The listing builds one solid part. Answer for the finished solid, in the listing's coordinates (mm). A direction names the side the tool comes from. Give positions to 0.01 mm unless a question says otherwise; leave off trailing zeros. Write each loop counter-clockwise with the first axis right and the second up, starting at its lowest first coordinate (ties: lowest second). Pieces come first, ordered by that corner, then holes. Notation, with made-up numbers: M 43.5,63.5 L 62.5,63.5 A15 cw 62.5,75.5 Z; hole C 60.25,73 d10. An arc over 180 degrees is marked long. Answer as a JSON object with one key per item and string values.
```python
from build123d import *

# Parameters (mm, degrees)
SKETCH_1_W                    = 20
SKETCH_1_H                    = 54.5
EXTRUDE_1_DEPTH               = 1
SKETCH_2_W                    = 20
SKETCH_2_H                    = 1
EXTRUDE_2_DEPTH               = 38
SKETCH_3_W                    = 20
SKETCH_3_H                    = 1
EXTRUDE_3_DEPTH               = 38
SKETCH_4_R                    = 4.1
CUT_EXTRUDE_1_DEPTH           = 1
SKETCH_5_R                    = 0.79
CUT_EXTRUDE_2_DEPTH           = 1
SKETCH_6_R                    = 0.79
CUT_EXTRUDE_3_DEPTH           = 1
SKETCH_7_R                    = 0.79
CUT_EXTRUDE_4_DEPTH           = 1
SKETCH_8_R                    = 0.79
CUT_EXTRUDE_5_DEPTH           = 1
SKETCH_9_R                    = 1.6
CUT_EXTRUDE_6_DEPTH           = 1
CUT_EXTRUDE_7_REACH           = 71.937
SKETCH_10_R                   = 1.6
CUT_EXTRUDE_8_REACH           = 71.937
SKETCH_11_R                   = 1.6
CUT_EXTRUDE_9_REACH           = 71.937
SKETCH_12_R                   = 1.6
CUT_EXTRUDE_10_REACH          = 71.937
SKETCH_14_R                   = 1.6
SHEET_START                   = -38
SHEET_METAL_1_OUTLINE_W       = 1
SHEET_METAL_1_OUTLINE_H       = 20
SHEET_METAL_1_DEPTH           = 38
SHEET_METAL_1_2_OUTLINE_W     = 37.35619449
SHEET_METAL_1_2_OUTLINE_H     = 20
SHEET_METAL_1_2_OUTLINE_R     = 0.79
SHEET_METAL_1_2_OUTLINE_R_2   = 4.1
SHEET_METAL_1_2_OUTLINE_R_3   = 1.6
SHEET_METAL_1_2_DEPTH         = 1
SHEET_START_2                 = 54.28876
SHEET_METAL_1_3_OUTLINE_W     = 1
SHEET_METAL_1_3_OUTLINE_H     = 20
SHEET_METAL_1_3_DEPTH         = 37.56743449
SHEET_START_3                 = -37.35619449
SHEET_METAL_1_3_2_OUTLINE_W   = 1
SHEET_METAL_1_3_2_OUTLINE_H   = 20
SHEET_METAL_1_3_2_DEPTH       = 37.55071449
SHEET_METAL_1_3_3_OUTLINE_R   = 4.1
SHEET_METAL_1_3_3_OUTLINE_R_2 = 1.6
SHEET_METAL_1_3_3_OUTLINE_R_3 = 0.79
SHEET_METAL_1_3_3_DEPTH       = 1
SHEET_METAL_1_3_4_OUTLINE_W   = 38
SHEET_METAL_1_3_4_OUTLINE_H   = 20
SHEET_METAL_1_3_4_OUTLINE_R   = 0.79
SHEET_METAL_1_3_4_OUTLINE_R_2 = 4.1
SHEET_METAL_1_3_4_DEPTH       = 2
SHEET_START_4                 = 52.5
SHEET_METAL_1_3_5_OUTLINE_W   = 38
SHEET_METAL_1_3_5_OUTLINE_H   = 20
SHEET_METAL_1_3_5_OUTLINE_R   = 0.79
SHEET_METAL_1_3_5_OUTLINE_R_2 = 4.1
SHEET_METAL_1_3_5_DEPTH       = 2
SHEET_START_5                 = -20
SHEET_METAL_1_3_6_DEPTH       = 20


with BuildPart() as part:
    # Sketch 1 → ﾎﾞｽ - 押し出し1 (new body)
    with BuildSketch(Plane(origin=(0, 0, 0), x_dir=(0, 0, -1), z_dir=(1, 0, 0))):
        with Locations((10, 27.25)):
            Rectangle(SKETCH_1_W, SKETCH_1_H)
    extrude(amount=EXTRUDE_1_DEPTH)

    # Sketch 2 → ﾎﾞｽ - 押し出し2 (add)
    with BuildSketch(Plane.ZY):
        with Locations((-10, 54)):
            Rectangle(SKETCH_2_W, SKETCH_2_H)
    extrude(amount=EXTRUDE_2_DEPTH)

    # ｽｹｯﾁ3 → ﾎﾞｽ - 押し出し3 (add)
    with BuildSketch(Plane.ZY):
        with Locations((-10, 0.5)):
            Rectangle(SKETCH_3_W, SKETCH_3_H)
    extrude(amount=EXTRUDE_3_DEPTH)

    # ｽｹｯﾁ4 → ｶｯﾄ - 押し出し1 (cut)
    with BuildSketch(Plane(origin=(0, 54.5, 0), x_dir=(1, 0, 0), z_dir=(0, 1, 0))):
        with Locations(Location((-26.39, 10, 0), (0, 0, 270))):
            Circle(SKETCH_4_R)
    extrude(amount=-CUT_EXTRUDE_1_DEPTH, mode=Mode.SUBTRACT)

    # ｽｹｯﾁ5 → ｶｯﾄ - 押し出し2 (cut)
    with BuildSketch(Plane(origin=(0, 54.5, 0), x_dir=(1, 0, 0), z_dir=(0, 1, 0))):
        with Locations(Location((-33.88, 10, 0), (0, 0, 270))):
            Circle(SKETCH_5_R)
    extrude(amount=-CUT_EXTRUDE_2_DEPTH, mode=Mode.SUBTRACT)

    # ｽｹｯﾁ6 → ｶｯﾄ - 押し出し3 (cut)
    with BuildSketch(Plane(origin=(0, 54.5, 0), x_dir=(1, 0, 0), z_dir=(0, 1, 0))):
        with Locations(Location((-18.9, 10, 0), (0, 0, 270))):
            Circle(SKETCH_6_R)
    extrude(amount=-CUT_EXTRUDE_3_DEPTH, mode=Mode.SUBTRACT)

    # ｽｹｯﾁ7 → ｶｯﾄ - 押し出し4 (cut)
    with BuildSketch(Plane(origin=(0, 54.5, 0), x_dir=(1, 0, 0), z_dir=(0, 1, 0))):
        with Locations(Location((-26.39, 2.51, 0), (0, 0, 270))):
            Circle(SKETCH_7_R)
    extrude(amount=-CUT_EXTRUDE_4_DEPTH, mode=Mode.SUBTRACT)

    # ｽｹｯﾁ8 → ｶｯﾄ - 押し出し5 (cut)
    with BuildSketch(Plane(origin=(0, 54.5, 0), x_dir=(1, 0, 0), z_dir=(0, 1, 0))):
        with Locations(Location((-26.39, 17.49, 0), (0, 0, 270))):
            Circle(SKETCH_8_R)
    extrude(amount=-CUT_EXTRUDE_5_DEPTH, mode=Mode.SUBTRACT)

    # ｽｹｯﾁ9 → ｶｯﾄ - 押し出し6 (cut)
    with BuildSketch(Plane(origin=(0, 0, 0), x_dir=(-1, 0, 0), z_dir=(0, -1, 0))):
        with Locations(Location((26.39, 10, 0), (0, 0, 90))):
            Circle(SKETCH_9_R)
    extrude(amount=-CUT_EXTRUDE_6_DEPTH, mode=Mode.SUBTRACT)

    # ｽｹｯﾁ10 → ｶｯﾄ - 押し出し7 (cut, up to next)
    with BuildSketch(Plane(origin=(1, 0, 0), x_dir=(0, 0, -1), z_dir=(1, 0, 0)), mode=Mode.PRIVATE) as cut_extrude_7_sk1:
        with Locations((17, 27.25)):
            Circle(SKETCH_10_R)
    cut_extrude_7_tool1 = extrude(cut_extrude_7_sk1.sketch, amount=-CUT_EXTRUDE_7_REACH, mode=Mode.PRIVATE) & part.part
    add(cut_extrude_7_tool1.solids().sort_by_distance((1, 27.25, -17))[0], mode=Mode.SUBTRACT)

    # ｽｹｯﾁ11 → ｶｯﾄ - 押し出し8 (cut, up to next)
    with BuildSketch(Plane(origin=(1, 0, 0), x_dir=(0, 0, -1), z_dir=(1, 0, 0)), mode=Mode.PRIVATE) as cut_extrude_8_sk1:
        with Locations((3, 27.25)):
            Circle(SKETCH_11_R)
    cut_extrude_8_tool1 = extrude(cut_extrude_8_sk1.sketch, amount=-CUT_EXTRUDE_8_REACH, mode=Mode.PRIVATE) & part.part
    add(cut_extrude_8_tool1.solids().sort_by_distance((1, 27.25, -3))[0], mode=Mode.SUBTRACT)

    # ｽｹｯﾁ12 → ｶｯﾄ - 押し出し9 (cut, up to next)
    with BuildSketch(Plane(origin=(1, 0, 0), x_dir=(0, 0, -1), z_dir=(1, 0, 0)), mode=Mode.PRIVATE) as cut_extrude_9_sk1:
        with Locations((10, 23.75)):
            Circle(SKETCH_12_R)
    cut_extrude_9_tool1 = extrude(cut_extrude_9_sk1.sketch, amount=-CUT_EXTRUDE_9_REACH, mode=Mode.PRIVATE) & part.part
    add(cut_extrude_9_tool1.solids().sort_by_distance((1, 23.75, -10))[0], mode=Mode.SUBTRACT)

    # ｽｹｯﾁ14 → ｶｯﾄ - 押し出し10 (cut, up to next)
    with BuildSketch(Plane(origin=(1, 0, 0), x_dir=(0, 0, -1), z_dir=(1, 0, 0)), mode=Mode.PRIVATE) as cut_extrude_10_sk1:
        with Locations((10, 30.75)):
            Circle(SKETCH_14_R)
    cut_extrude_10_tool1 = extrude(cut_extrude_10_sk1.sketch, amount=-CUT_EXTRUDE_10_REACH, mode=Mode.PRIVATE) & part.part
    add(cut_extrude_10_tool1.solids().sort_by_distance((1, 30.75, -10))[0], mode=Mode.SUBTRACT)

    # Sheet Metal 1: read off the stored shape, not the designer's step
    # Sheet Metal 1 outline → Sheet Metal 1 (cut)
    with BuildSketch(Plane.YZ.offset(SHEET_START)):
        with Locations((54, -10)):
            Rectangle(SHEET_METAL_1_OUTLINE_W, SHEET_METAL_1_OUTLINE_H)
        with Locations((0.5, -10)):
            Rectangle(SHEET_METAL_1_OUTLINE_W, SHEET_METAL_1_OUTLINE_H)
    extrude(amount=SHEET_METAL_1_DEPTH, mode=Mode.SUBTRACT)

    # Sheet Metal 1 2 outline → Sheet Metal 1 2 (add)
    # profile 1 of 2: a face of its own
    with BuildSketch(Plane.YZ):
        with Locations((73.178097245, -10)):
            Rectangle(SHEET_METAL_1_2_OUTLINE_W, SHEET_METAL_1_2_OUTLINE_H)
        with Locations((80.24619449, -17.49)):
            Circle(SHEET_METAL_1_2_OUTLINE_R, mode=Mode.SUBTRACT)
        with Locations((72.75619449, -10)):
            Circle(SHEET_METAL_1_2_OUTLINE_R, mode=Mode.SUBTRACT)
        with Locations((80.24619449, -10)):
            Circle(SHEET_METAL_1_2_OUTLINE_R_2, mode=Mode.SUBTRACT)
        with Locations((87.73619449, -10)):
            Circle(SHEET_METAL_1_2_OUTLINE_R, mode=Mode.SUBTRACT)
        with Locations((80.24619449, -2.51)):
            Circle(SHEET_METAL_1_2_OUTLINE_R, mode=Mode.SUBTRACT)
    # profile 2 of 2: a face of its own
    with BuildSketch(Plane.YZ):
        with Locations((-18.678097245, -10)):
            Rectangle(SHEET_METAL_1_2_OUTLINE_W, SHEET_METAL_1_2_OUTLINE_H)
        with Locations((-25.74619449, -10)):
            Circle(SHEET_METAL_1_2_OUTLINE_R_3, mode=Mode.SUBTRACT)
    extrude(amount=SHEET_METAL_1_2_DEPTH)

    # Sheet Metal 1 3: read off the stored shape, not the designer's step
    # Sheet Metal 1 3 outline → Sheet Metal 1 3 (cut)
    with BuildSketch(Plane(origin=(0, 0, 0), x_dir=(1, 0, 0), z_dir=(0, 1, 0)).offset(SHEET_START_2)):
        with Locations((0.5, 10)):
            Rectangle(SHEET_METAL_1_3_OUTLINE_W, SHEET_METAL_1_3_OUTLINE_H)
    extrude(amount=SHEET_METAL_1_3_DEPTH, mode=Mode.SUBTRACT)

    # Sheet Metal 1 3 2 outline → Sheet Metal 1 3 2 (cut)
    with BuildSketch(Plane(origin=(0, 0, 0), x_dir=(1, 0, 0), z_dir=(0, 1, 0)).offset(SHEET_START_3)):
        with Locations((0.5, 10)):
            Rectangle(SHEET_METAL_1_3_2_OUTLINE_W, SHEET_METAL_1_3_2_OUTLINE_H)
    extrude(amount=SHEET_METAL_1_3_2_DEPTH, mode=Mode.SUBTRACT)



with BuildPart() as body_2:
    # Sheet Metal 1 3 3 outline → Sheet Metal 1 3 3 (new body)
    # profile 1 of 5: a face of its own
    with BuildSketch(Plane(origin=(0, 0, 0), x_dir=(1, 0, 0), z_dir=(0, 1, 0))):
        with Locations((-26.39, 10)):
            Circle(SHEET_METAL_1_3_3_OUTLINE_R)
        with Locations((-26.39, 10)):
            Circle(SHEET_METAL_1_3_3_OUTLINE_R_2, mode=Mode.SUBTRACT)
    # profile 2 of 5: a face of its own
    with BuildSketch(Plane(origin=(0, 0, 0), x_dir=(1, 0, 0), z_dir=(0, 1, 0))):
        with Locations((-33.88, 10)):
            Circle(SHEET_METAL_1_3_3_OUTLINE_R_3)
    # profile 3 of 5: a face of its own
    with BuildSketch(Plane(origin=(0, 0, 0), x_dir=(1, 0, 0), z_dir=(0, 1, 0))):
        with Locations((-18.9, 10)):
            Circle(SHEET_METAL_1_3_3_OUTLINE_R_3)
    # profile 4 of 5: a face of its own
    with BuildSketch(Plane(origin=(0, 0, 0), x_dir=(1, 0, 0), z_dir=(0, 1, 0))):
        with Locations((-26.39, 2.51)):
            Circle(SHEET_METAL_1_3_3_OUTLINE_R_3)
    # profile 5 of 5: a face of its own
    with BuildSketch(Plane(origin=(0, 0, 0), x_dir=(1, 0, 0), z_dir=(0, 1, 0))):
        with Locations((-26.39, 17.49)):
            Circle(SHEET_METAL_1_3_3_OUTLINE_R_3)
    extrude(amount=SHEET_METAL_1_3_3_DEPTH)


with BuildPart() as part_1:
    add(part.part)

    add(body_2.part)  # Sheet Metal 1 3 4 merges body 2
    # Sheet Metal 1 3 4 outline → Sheet Metal 1 3 4 (add)
    with BuildSketch(Plane(origin=(0, 0, 0), x_dir=(1, 0, 0), z_dir=(0, 1, 0))):
        with Locations((-19, 10)):
            Rectangle(SHEET_METAL_1_3_4_OUTLINE_W, SHEET_METAL_1_3_4_OUTLINE_H)
        with Locations((-26.39, 2.51)):
            Circle(SHEET_METAL_1_3_4_OUTLINE_R, mode=Mode.SUBTRACT)
        with Locations((-33.88, 10)):
            Circle(SHEET_METAL_1_3_4_OUTLINE_R, mode=Mode.SUBTRACT)
        with Locations((-26.39, 10)):
            Circle(SHEET_METAL_1_3_4_OUTLINE_R_2, mode=Mode.SUBTRACT)
        with Locations((-18.9, 10)):
            Circle(SHEET_METAL_1_3_4_OUTLINE_R, mode=Mode.SUBTRACT)
        with Locations((-26.39, 17.49)):
            Circle(SHEET_METAL_1_3_4_OUTLINE_R, mode=Mode.SUBTRACT)
    extrude(amount=SHEET_METAL_1_3_4_DEPTH)

    # Sheet Metal 1 3 5 outline → Sheet Metal 1 3 5 (add)
    with BuildSketch(Plane(origin=(0, 0, 0), x_dir=(1, 0, 0), z_dir=(0, 1, 0)).offset(SHEET_START_4)):
        with Locations((-19, 10)):
            Rectangle(SHEET_METAL_1_3_5_OUTLINE_W, SHEET_METAL_1_3_5_OUTLINE_H)
        with Locations((-26.39, 2.51)):
            Circle(SHEET_METAL_1_3_5_OUTLINE_R, mode=Mode.SUBTRACT)
        with Locations((-33.88, 10)):
            Circle(SHEET_METAL_1_3_5_OUTLINE_R, mode=Mode.SUBTRACT)
        with Locations((-26.39, 10)):
            Circle(SHEET_METAL_1_3_5_OUTLINE_R_2, mode=Mode.SUBTRACT)
        with Locations((-18.9, 10)):
            Circle(SHEET_METAL_1_3_5_OUTLINE_R, mode=Mode.SUBTRACT)
        with Locations((-26.39, 17.49)):
            Circle(SHEET_METAL_1_3_5_OUTLINE_R, mode=Mode.SUBTRACT)
    extrude(amount=SHEET_METAL_1_3_5_DEPTH)

    # Sheet Metal 1 3 6 outline → Sheet Metal 1 3 6 (cut)
    with BuildSketch(Plane.XY.offset(SHEET_START_5)):
        with BuildLine():
            Line((-38, 2), (-38, 1))
            Line((-38, 1), (-1, 1))
            ThreePointArc((-1, 1), (-0.292893219, 1.292893219), (0, 2))
            Line((0, 2), (-38, 2))
        make_face()
        with BuildLine():
            Line((-1, 53.5), (-38, 53.5))
            Line((-38, 53.5), (-38, 52.5))
            Line((-38, 52.5), (0, 52.5))
            ThreePointArc((0, 52.5), (-0.292893219, 53.207106781), (-1, 53.5))
        make_face()
        with BuildLine():
            ThreePointArc((-1, 54.5), (0.414213562, 53.914213562), (1, 52.5))
            Line((1, 52.5), (1, 54.28876))
            Line((1, 54.28876), (0, 54.28876))
            Line((0, 54.28876), (0, 54.5))
            Line((0, 54.5), (-1, 54.5))
        make_face()
        with BuildLine():
            ThreePointArc((1, 2), (0.414213562, 0.585786438), (-1, 0))
            Line((-1, 0), (0, 0))
            Line((0, 0), (0, 0.19452))
            Line((0, 0.19452), (1, 0.19452))
            Line((1, 0.19452), (1, 2))
        make_face()
    extrude(amount=SHEET_METAL_1_3_6_DEPTH, mode=Mode.SUBTRACT)


solid = part_1.part
```
1. Consider line 1 along Z through (x, y) = (-26.39, 54.15); line 2 along Y through (x, z) = (-36, -6.5); line 3 along X through (y, z) = (49, -7). Determine where each line is inside the solid, lowest interval first.
Verdict:
{"line 1": "z = -20 to -18.28, -16.7 to -14.1, -5.9 to -3.3, -1.72 to 0", "line 2": "y = 0 to 1, 53.5 to 54.5", "line 3": "x = 0 to 1"}
2. A cutting plane is placed at A-A, the plane x = -21.5. Give the vertices of the cut face in (y, z).
Verdict:
{"outline": "M 0,-20 L 1,-20 L 1,0 L 0,0 Z; M 53.5,-20 L 54.5,-20 L 54.5,0 L 53.5,0 Z"}
3. A flat-ended cylindrical pin translates along its axis: pin 1 (8 mm diameter, centred on y = 38, z = -10.5, fed in from -X). Find the tip coordinate at first contact, or state that the pin passes through.
Verdict:
{"pin 1": "stops at x = 0"}
4. A cutting plane is placed at D-D, the plane y = 26.5. Give the vertices of the cut face in (x, z), plus the area to 3 significant figures.
Verdict:
{"outline": "M 0,-20 L 1,-20 L 1,-18.41 L 0,-18.41 Z; M 0,-15.59 L 1,-15.59 L 1,-4.41 L 0,-4.41 Z; M 0,-1.59 L 1,-1.59 L 1,0 L 0,0 Z", "area": "14.3 mm2"}
5. For faces 1 (the cylindrical face through (-24.91, 0.49, -9.39)), 2 (the cylindrical face through (-22.603, 53.993, -8.43)), 3 (the flat face through (-20, 1, -10)), determine the directions among +Z, -Z, +X, -X, +Y, -Y from which every point of the face is accessible in a straight line to the end or side of a thin tool.
Verdict:
{"face 1": "+Y, -Y", "face 2": "+Y", "face 3": "+Z, -Z, -X"}
6. The mould has two halves that part along Y. Classify faces 4 (the cylindrical face through (-25.636, 53.993, -17.727)), 5 (the flat face through (-20, 0, -10)), 6 (the flat face through (-19, 53.5, -12)), 7 (the flat face through (0, 27, -10)): released by +Y, released by -Y, zero draft, split by the parting line, or undercut.
Verdict:
{"face 4": "zero draft", "face 5": "released by -Y", "face 6": "undercut", "face 7": "undercut"}
7. A cutting plane is placed at C-C, the plane z = -13.5. Give the vertices of the cut face in (x, y), plus the area to 3 significant figures.
Verdict:
{"outline": "M -38,0 L -1,0 A2 ccw 1,2 L 1,52.5 A2 ccw -1,54.5 L -24.25,54.5 L -24.25,53.5 L -1,53.5 A1 cw 0,52.5 L 0,2 A1 cw -1,1 L -38,1 Z; M -38,53.5 L -28.53,53.5 L -28.53,54.5 L -38,54.5 Z", "area": "125 mm2"}
8. A cutting plane is placed at B-B, the plane x = -33.88. Give the vertices of the cut face in (y, z), plus the area to 3 significant figures.
Verdict:
{"outline": "M 0,-20 L 1,-20 L 1,0 L 0,0 Z; M 53.5,-20 L 54.5,-20 L 54.5,-10.79 L 53.5,-10.79 Z; M 53.5,-9.21 L 54.5,-9.21 L 54.5,0 L 53.5,0 Z", "area": "38.4 mm2"}
